Verification items for the finished model (mm, model axes). A direction names the side the tool comes from. Coordinates: 2 decimals unless noted, no trailing zeros. Write each loop counter-clockwise with the first axis right and the second up, starting at its lowest first coordinate (ties: lowest second). Pieces come first, ordered by that corner, then holes. Notation, with made-up numbers: (-35, -29) - (-31, -29) arc R13 cw to (-31, -23) - close; hole circle Ø3 at (69.5, -30). An arc over 180 degrees is marked (long way). Answer as CSV lines item,"result". Start each with the question number.
```python
from build123d import *

# Parameters (mm, degrees)
F0_W     = 368.3
F0_H     = 25.4
F1_DEPTH = 12.7
F2_W     = 6.35
F2_H     = 6.35
F3_DEPTH = 368.301
F5_DEPTH = 25.401
F6_W     = 6.35
F6_H     = 6.35
F7_DEPTH = 260.428428
F8_W     = 6.35
F8_H     = 6.35
F9_DEPTH = 260.428428


with BuildPart() as f1:
    # F0 (on Front) → F1 (new body)
    with BuildSketch(Plane.XZ):
        with Locations((0, 12.7)):
            Rectangle(F0_W, F0_H)
    extrude(amount=F1_DEPTH)

    # F2 (on face) → F3 (cut, through all)
    with BuildSketch(Plane.YZ.offset(184.15)):
        with Locations((-3.175, 15.875)):
            Rectangle(F2_W, F2_H)
    extrude(amount=-F3_DEPTH, mode=Mode.SUBTRACT)

    # F4 (on face) → F5 (cut, through all)
    with BuildSketch(Plane.XY.offset(25.4)):
        Polygon((-171.45, 0), (-184.15, 0), (-184.15, -12.7), align=None)
        Polygon((171.45, 0), (184.15, -12.7), (184.15, 0), align=None)
    extrude(amount=-F5_DEPTH, mode=Mode.SUBTRACT)

    # F6 (on face) → F7 (cut, through all)
    with BuildSketch(Plane(origin=(85.725, 85.725, 0), x_dir=(-0.707107, 0.707107, 0), z_dir=(0.707107, 0.707107, 0))):
        with Locations((-136.01897, 12.7)):
            Rectangle(F6_W, F6_H)
    extrude(amount=-F7_DEPTH, mode=Mode.SUBTRACT)

    # F8 (on face) → F9 (cut, through all)
    with BuildSketch(Plane(origin=(-85.725, 85.725, 0), x_dir=(-0.707107, -0.707107, 0), z_dir=(-0.707107, 0.707107, 0))):
        with Locations((136.01897, 12.7)):
            Rectangle(F8_W, F8_H)
    extrude(amount=-F9_DEPTH, mode=Mode.SUBTRACT)


solid = f1.part
```
1. Scan lines: line 1 along Z through (x, y) = (43, -4.25); line 2 along Y through (x, z) = (-168, 14.75); line 3 along X through (y, z) = (-3.75, 11.25). Record each from-to range of solid material in increasing order. Write a range as from..to.
2. Cross-section at A-A (y = -4). Record the cut outline in (x, z).
3. Access from +Z, -Z, +X, -X, +Y, -Y to the whole of each face (thin tool, end or side, straight path). Record for faces 1 (the face through (2, -3, 12.7)), 2 (the face through (-3, -12.7, 13)).
4. Draft check along Z on faces 3 (the face through (-179.3, -7.85, 12.88)), 4 (the face through (2, -6.35, 16)), 5 (the face through (-3, -6, 25.4)). Enter one of: pulls with the +Z half, pulls with the -Z half, needs draft (parallel to the pull), parting line crosses it, or undercut.
5. Cross-section at C-C (z = 5). Record the cut outline in (x, y).
6. Cross-section at B-B (x = -99.5). Record the cut outline in (y, z), and give its area (3 significant figures).
7. Depth check by flat-ended pin: P1, Ø12, axis at x = 88.5, z = 8, coming from the +Y side; P2, Ø4, axis at y = -10, z = 17.5, coming from the +X side; P3, Ø5, axis at x = -64.5, z = 15.5, coming from the +Y side; P4, Ø3, axis at y = -9.5, z = 14, coming from the +X side. Enter the tip coordinate at first touch or a pass-through.
Completed:
1,line 1,"z = 0..12.7, 19.05..25.4"
1,line 2,"y = -12.7..-6.35"
1,line 3,"x = -175.2..175.2"
2,outline,"(-175.45, 0) - (175.45, 0) - (175.45, 12.7) - (-175.45, 12.7) - close; (-175.45, 19.05) - (175.45, 19.05) - (175.45, 25.4) - (-175.45, 25.4) - close"
3,face 1,"+X, -X, +Y"
3,face 2,"+Z, -Z, +X, -X, -Y"
4,face 3,"needs draft"
4,face 4,"undercut"
4,face 5,"pulls with the +Z half"
5,outline,"(-184.15, -12.7) - (184.15, -12.7) - (171.45, 0) - (-171.45, 0) - close"
6,outline,"(-12.7, 0) - (0, 0) - (0, 12.7) - (-6.35, 12.7) - (-6.35, 19.05) - (0, 19.05) - (0, 25.4) - (-12.7, 25.4) - close"
6,area,"282 mm2"
7,P1,"stops at y = 0"
7,P2,"stops at x = 183.45"
7,P3,"stops at y = -6.35"
7,P4,"stops at x = 179.66"
